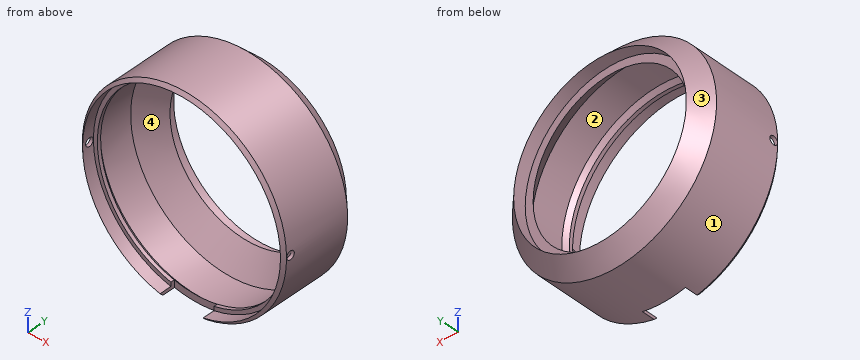
```python
from build123d import *

# Parameters (mm, degrees)
SKETCH2_W               = 10.9
SKETCH2_H               = 4.3
CUT_EXTRUDE1_DEPTH      = 26.9
SKETCH3_R               = 1.05
CUT_EXTRUDE2_DEPTH      = 26.9
CUT_EXTRUDE2_DEPTH_BACK = 26.9


with BuildPart() as part:
    # Sketch1 → Revolve1 (revolve)
    with BuildSketch(Plane.XY):
        Polygon((25.1, 1), (24.1, 0), (24.1, -0.9), (25.1, -0.9), (25.1, -3.9), (25.9, -3.1), (25.9, 13.8), (21.9, 17.8), (21.9, 14.6), (19.9, 14.6), (25.1, 9.4), align=None)
    revolve(axis=Axis((0, -5, 0), (0, 1, 0)))

    # Sketch2 → Cut-Extrude1 (cut, through all)
    with BuildSketch(Plane.XY):
        with Locations((0, -2.05)):
            Rectangle(SKETCH2_W, SKETCH2_H)
    extrude(amount=-CUT_EXTRUDE1_DEPTH, mode=Mode.SUBTRACT)

    # Sketch3 → Cut-Extrude2 (cut, two sides)
    with BuildSketch(Plane(origin=(0, 0, 0), x_dir=(0, 0, -1), z_dir=(1, 0, 0))) as cut_extrude2_sk:
        with Locations((0, -2)):
            Circle(SKETCH3_R)
    extrude(amount=CUT_EXTRUDE2_DEPTH, mode=Mode.SUBTRACT)
    extrude(cut_extrude2_sk.sketch, amount=-CUT_EXTRUDE2_DEPTH_BACK, mode=Mode.SUBTRACT)


solid = part.part
```
The model under review builds one solid part; all positions refer to its coordinate system, in mm. Face numbers are marked on the shaded views. A direction names the side the tool comes from. Give positions to 0.01 mm unless a question says otherwise; leave off trailing zeros. Write each loop counter-clockwise with the first axis right and the second up, starting at its lowest first coordinate (ties: lowest second). Pieces come first, ordered by that corner, then holes. Notation, with made-up numbers: M 88,13 L 124,13 A28 cw 124,39 Z; hole C 51,-14.5 d1. An arc over 180 degrees is marked long. Answer in a Markdown table with one row per item.
Item 1: Add section C-C on y = 15.5. Give the boundary of the cut face in (x, z).
Check sheet entries:
| item | result |
|---|---|
| outline | C 0,0 d48.4; hole C 0,0 d43.8 |
Item 2: Add section D-D on y = 6.5. Give the boundary of the cut face in (x, z), plus the area to 3 significant figures.
Check sheet entries:
| item | result |
|---|---|
| outline | C 0,0 d51.8; hole C 0,0 d50.2 |
| area | 128 mm2 |
Item 3: Draft analysis for pull direction Y (two halves, no side actions). For the marked faces 3 and 4, state which applies: +Y half, -Y half, draft (parallel to the pull), parting line (faces both ways), or undercut.
Check sheet entries:
| item | result |
|---|---|
| face 3 | +Y half |
| face 4 | undercut |
Item 4: Add section B-B on z = 0. State how many separate pieces and enclosed holes the cut face has, plus the area to 3 significant figures.
Check sheet entries:
| item | result |
|---|---|
| separate pieces | 4 |
| enclosed holes | 0 |
| area | 65.0 mm2 |
Item 5: For P1, Ø5, axis at x = 10, y = 14, coming from the +Z side; P2, Ø1.5, axis at x = 3, y = 7.5, coming from the -Z side; P3, Ø1.2, axis at x = 1, z = -25, coming from the -Y side; P4, Ø1.7, axis at y = -2, z = 0, coming from the +X side, all flat-tipped, find the tip position at first contact; note any pin that passes through.
Check sheet entries:
| item | result |
|---|---|
| P1 | z = 24.79 |
| P2 | z = -25.8 |
| P3 | y = 0.1 |
| P4 | through |
Item 6: Tool access review of the marked faces 1 and 2: name each direction out of +Z, -Z, +X, -X, +Y, -Y from which nothing blocks a thin tool from reaching the whole face with its end or side.
Check sheet entries:
| item | result |
|---|---|
| face 1 | +Y, -Y |
| face 2 | none |
Item 7: For line 1 along Z through (x, y) = (0, 5.25); line 2 along X through (y, z) = (-2.25, -22.5); line 3 along Z through (x, y) = (0, 16.05), list the stretches that pass through material, from the lowest coordinate up.
Check sheet entries:
| item | result |
|---|---|
| line 1 | -25.9 to -25.1, 25.1 to 25.9 |
| line 2 | -12.83 to -11.12, 11.12 to 12.83 |
| line 3 | -23.65 to -21.9, 21.9 to 23.65 |
Item 8: Add section A-A on x = 0. Give the boundary of the cut face in (y, z), plus the area to 3 significant figures.
Check sheet entries:
| item | result |
|---|---|
| outline | M -3.9,25.1 L -0.9,25.1 L -0.9,24.1 L 0,24.1 L 1,25.1 L 9.4,25.1 L 14.6,19.9 L 14.6,21.9 L 17.8,21.9 L 13.8,25.9 L -3.1,25.9 Z; M 0.1,-25.9 L 13.8,-25.9 L 17.8,-21.9 L 14.6,-21.9 L 14.6,-19.9 L 9.4,-25.1 L 1,-25.1 L 0.1,-24.2 Z |
| area | 64.5 mm2 |
